```python
from build123d import *

# Parameters (mm, degrees)
BOSS_EXTRUDE1_DEPTH = 3.302
SKETCH2_R           = 3.302
CUT_EXTRUDE1_DEPTH  = 23.368


with BuildPart() as part:
    # Sketch1 → Boss-Extrude1 (new body)
    with BuildSketch(Plane(origin=(0, 0, 0), x_dir=(1, 0, 0), z_dir=(0, 1, 0))):
        Polygon((0, 0), (-48.26, 0), (-101.346, 61.976), (-101.346, 137.16), (0, 137.16), align=None)
    extrude(amount=BOSS_EXTRUDE1_DEPTH)

    # Sketch2 → Cut-Extrude1 (cut)
    with BuildSketch(Plane(origin=(0, 3.302, 0), x_dir=(1, 0, 0), z_dir=(0, 1, 0))):
        with Locations(Location((-93.726, 70.612, 0), (0, 0, 270))):
            Circle(SKETCH2_R)
        with Locations(Location((-24.892, 13.462, 0), (0, 0, 270))):
            Circle(SKETCH2_R)
        with Locations(Location((-6.604, 70.612, 0), (0, 0, 270))):
            Circle(SKETCH2_R)
        with Locations(Location((-6.604, 130.556, 0), (0, 0, 270))):
            Circle(SKETCH2_R)
        with Locations(Location((-93.726, 130.556, 0), (0, 0, 270))):
            Circle(SKETCH2_R)
    extrude(amount=-CUT_EXTRUDE1_DEPTH, mode=Mode.SUBTRACT)


solid = part.part
```
Input: part model. Units: mm. Frame: model coordinates. Coordinates: 2 decimals unless noted, no trailing zeros. Order: outer loops, then holes, each group sorted by start corner. A loop starts at its lowest first (then second) coordinate and runs counter-clockwise, first axis right, second up. Notation, with made-up numbers: (68, 23.25) - (104, 23.25) arc R19 ccw to (104, 52.25) - close; hole circle Ø7 at (-37, 88). An arc over 180 degrees is marked (long way). Return JSON: item names as keys, results as strings.
Q1. Cut plane B-B (y = 2.55). Return loops of the section in (x, z).
The answers:
{"outline": "(-101.35, -137.16) - (0, -137.16) - (0, 0) - (-48.26, 0) - (-101.35, -61.98) - close; hole circle Ø6.6 at (-93.73, -130.56); hole circle Ø6.6 at (-93.73, -70.61); hole circle Ø6.6 at (-24.89, -13.46); hole circle Ø6.6 at (-6.6, -130.56); hole circle Ø6.6 at (-6.6, -70.61)"}
Q2. First-contact query: pin 1 (8.5 mm diameter, centred on x = -6.604, z = -130.556, fed in from -Y); pin 2 (4 mm diameter, centred on x = -93.726, z = -130.556, fed in from +Y). Flat tips, straight axial feed; report the tip coordinate or a pass-through.
The answers:
{"pin 1": "stops at y = 0", "pin 2": "passes through"}
Q3. Cut plane A-A (z = -14). Return loops of the section in (x, y), then the cut area to 3 significant figures.
The answers:
{"outline": "(-60.25, 0) - (-28.15, 0) - (-28.15, 3.3) - (-60.25, 3.3) - close; (-21.63, 0) - (0, 0) - (0, 3.3) - (-21.63, 3.3) - close", "area": "177 mm2"}
Q4. Ray query, probe 1 along Z at (x, y) = (-5.5, 2.15); probe 2 along Z at (x, y) = (-96.5, 1.15); probe 3 along X at (y, z) = (0.2, -14.5). Return the intervals inside material, ascending.
The answers:
{"probe 1": "z = -137.16 to -133.67, -127.44 to -73.72, -67.5 to 0", "probe 2": "z = -137.16 to -132.35, -128.76 to -72.4, -68.82 to -56.32", "probe 3": "x = -60.68 to -28.03, -21.76 to 0"}
Q5. Cut plane D-D (z = -40.5). Return loops of the section in (x, y).
The answers:
{"outline": "(-82.95, 0) - (0, 0) - (0, 3.3) - (-82.95, 3.3) - close"}
Q6. Draft query along Z for faces 1 (the flat face through (-51, 2, -137.16)), 2 (the cylindrical face through (-94.991, 1.674, -127.506)), 3 (the flat face through (-74.43, 1.63, -30.55)), 4 (the flat face through (-50, 3.302, -70)). Return one class per face: +Z half, -Z half, draft (parallel to the pull), parting line (faces both ways), or undercut.
The answers:
{"face 1": "-Z half", "face 2": "undercut", "face 3": "+Z half", "face 4": "draft"}
Q7. Cut plane C-C (x = -69). Return loops of the section in (y, z), then the cut area to 3 significant figures.
The answers:
{"outline": "(0, -137.16) - (3.3, -137.16) - (3.3, -24.21) - (0, -24.21) - close", "area": "373 mm2"}
